```python
from build123d import *

# Parameters (mm, degrees)
SKETCH4_W           = 53
SKETCH4_H           = 53
BOSS_EXTRUDE3_DEPTH = 2
FILLET1_R           = 2


with BuildPart() as part:
    # Sketch1 → Loft2 section 0
    with BuildSketch(Plane(origin=(0, 0, 0), x_dir=(1, 0, 0), z_dir=(0, 1, 0))):
        with BuildLine():
            Line((-26.5, -26.5), (26.5, -26.5))
            Line((26.5, -26.5), (26.5, 26.5))
            Line((26.5, 26.5), (-26.5, 26.5))
            Line((-26.5, 26.5), (-26.5, -26.5))
        make_face()
    # Sketch3 → Loft2 section 1
    with BuildSketch(Plane(origin=(0, 25, 0), x_dir=(1, 0, 0), z_dir=(0, 1, 0))):
        with BuildLine():
            Line((-29.5, 29.5), (29.5, 29.5))
            Line((29.5, 29.5), (29.5, -29.5))
            Line((29.5, -29.5), (-29.5, -29.5))
            Line((-29.5, -29.5), (-29.5, 29.5))
        make_face()
    loft()

    # Sketch1<198> → Cut-Loft1 section 0
    with BuildSketch(Plane(origin=(0, 0, 0), x_dir=(1, 0, 0), z_dir=(0, 1, 0))):
        with BuildLine():
            Line((-24.5, 24.5), (24.5, 24.5))
            Line((24.5, 24.5), (24.5, -24.5))
            Line((24.5, -24.5), (-24.5, -24.5))
            Line((-24.5, -24.5), (-24.5, 24.5))
        make_face()
    # Sketch3<140> → Cut-Loft1 section 1
    with BuildSketch(Plane(origin=(0, 25, 0), x_dir=(1, 0, 0), z_dir=(0, 1, 0))):
        with BuildLine():
            Line((-27.5, -27.5), (27.5, -27.5))
            Line((27.5, -27.5), (27.5, 27.5))
            Line((27.5, 27.5), (-27.5, 27.5))
            Line((-27.5, 27.5), (-27.5, -27.5))
        make_face()
    loft(mode=Mode.SUBTRACT)

    # Sketch4 → Boss-Extrude3 (add)
    with BuildSketch(Plane.XZ):
        Rectangle(SKETCH4_W, SKETCH4_H)
    extrude(amount=-BOSS_EXTRUDE3_DEPTH)

    # Fillet1
    fillet1_edges = [part.edges().sort_by_distance(p)[0] for p in [
        (-26.12, 13.5, 26.12),
        (-26.12, 13.5, -26.12),
        (26.12, 13.5, 26.12),
        (26.12, 13.5, -26.12),
        (28, 12.5, 28),
        (-28, 12.5, 28),
        (-28, 12.5, -28),
        (28, 12.5, -28),
        (0, 0, 26.5),
        (-26.5, 0, 0),
        (26.5, 0, 0),
        (0, 0, -26.5),
    ]]
    fillet(fillet1_edges, radius=FILLET1_R)


solid = part.part
```
Model file for the job. Use its own axes, mm. Coordinates: 2 decimals unless noted, no trailing zeros. Use a Markdown table: item, result. Add a question column.
Item 1: Drop flat-ended pins along their axis: pin 1 (12 mm diameter, centred on x = -1.5, z = 18, fed in from -Y); pin 2 (10 mm diameter, centred on y = 21.5, z = 10.5, fed in from -X); pin 3 (1.5 mm diameter, centred on y = 7.5, z = 5.5, fed in from -X); pin 4 (1 mm diameter, centred on y = 14.5, z = 16, fed in from -X). Give the stop position or say it passes through.
Item 2: Drill centre lines: line 1 along Z through (x, y) = (-25.5, 13.5); line 2 along Z through (x, y) = (22.5, 22); line 3 along X through (y, z) = (13.25, -10.5). Where is each one in solid material? Low to high.
Item 3: Two-plate mould, pull along Z, no slides. Class faces 1 (the face through (0, 2, 0)), 2 (the face through (0, 0, 1)): pulls with the +Z half, pulls with the -Z half, needs draft (parallel to the pull), parting line crosses it, or undercut.
A:
| question | item | result |
|---|---|---|
| 1 | pin 1 | stops at y = 0 |
| 1 | pin 2 | stops at x = -29.5 |
| 1 | pin 3 | stops at x = -27.49 |
| 1 | pin 4 | stops at x = -28.3 |
| 2 | line 1 | z = -28.12 to -25.58, 25.58 to 28.12 |
| 2 | line 2 | z = -29.14 to -27.14, 27.14 to 29.14 |
| 2 | line 3 | x = -28.09 to -26.09, 26.09 to 28.09 |
| 3 | face 1 | undercut |
| 3 | face 2 | needs draft |
